Could you check a few things on this model? Use its own coordinates, in mm. Coordinates: 2 decimals unless noted, no trailing zeros. Order: outer loops, then holes, each group sorted by start corner. A loop starts at its lowest first (then second) coordinate and runs counter-clockwise, first axis right, second up. Notation, with made-up numbers: (79, -18.5) - (107, -18.5) arc R20 ccw to (107, 20.5) - close; hole circle Ø8 at (53.25, 63). An arc over 180 degrees is marked (long way). One line per item, written item: value.
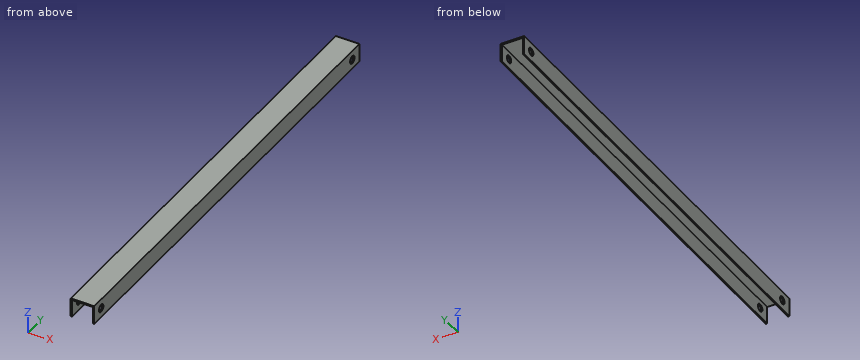
from build123d import *

# Parameters (mm, degrees)
BOSS_EXTRUDE1_DEPTH      = 145
BOSS_EXTRUDE1_DEPTH_BACK = 145
SKETCH1_W                = 15
SKETCH1_H                = 12
CUT_EXTRUDE1_DEPTH       = 200
CUT_EXTRUDE1_DEPTH_BACK  = 200
SKETCH2_W                = 13.28
SKETCH2_H                = 14
CUT_EXTRUDE2_DEPTH       = 200
CUT_EXTRUDE2_DEPTH_BACK  = 200
SKETCH3_R                = 2.4


with BuildPart() as part:
    # Sketch1 → Boss-Extrude1 (new, two sides: drawn at the far end of the back side and taken through both)
    with BuildSketch(Plane(origin=(0, 0, 0), x_dir=(1, 0, 0), z_dir=(0, 1, 0)).offset(-BOSS_EXTRUDE1_DEPTH_BACK)):
        Rectangle(SKETCH1_W, SKETCH1_H)
    extrude(amount=BOSS_EXTRUDE1_DEPTH + BOSS_EXTRUDE1_DEPTH_BACK)

    # Sketch2 → Cut-Extrude1 (cut, two sides: drawn at the far end of the back side and taken through both)
    with BuildSketch(Plane(origin=(0, 0, 0), x_dir=(1, 0, 0), z_dir=(0, 1, 0)).offset(-CUT_EXTRUDE1_DEPTH_BACK)):
        with Locations((0, 1.86)):
            Rectangle(SKETCH2_W, SKETCH2_H)
    extrude(amount=CUT_EXTRUDE1_DEPTH + CUT_EXTRUDE1_DEPTH_BACK, mode=Mode.SUBTRACT)

    # Sketch3 → Cut-Extrude2 (cut, two sides: drawn at the far end of the back side and taken through both)
    with BuildSketch(Plane(origin=(0, 0, 0), x_dir=(0, 0, -1), z_dir=(1, 0, 0)).offset(-CUT_EXTRUDE2_DEPTH_BACK)):
        with Locations(Location((0, 137.33, 0), (0, 0, 180))):
            Circle(SKETCH3_R)
        with Locations(Location((0, -137.33, 0), (0, 0, 180))):
            Circle(SKETCH3_R)
    extrude(amount=CUT_EXTRUDE2_DEPTH + CUT_EXTRUDE2_DEPTH_BACK, mode=Mode.SUBTRACT)


solid = part.part
Item 1: I want a section at C-C on x = -1.75. Please give me the cut outline in (y, z).
Conclusion:
outline: (-145, 5.14) - (145, 5.14) - (145, 6) - (-145, 6) - close
Item 2: I want a section at B-B on z = 0. Please give me the cut outline in (x, y).
Conclusion:
outline: (-7.5, -145) - (-6.64, -145) - (-6.64, -139.73) - (-7.5, -139.73) - close; (-7.5, -134.93) - (-6.64, -134.93) - (-6.64, 134.93) - (-7.5, 134.93) - close; (-7.5, 139.73) - (-6.64, 139.73) - (-6.64, 145) - (-7.5, 145) - close; (6.64, -145) - (7.5, -145) - (7.5, -139.73) - (6.64, -139.73) - close; (6.64, -134.93) - (7.5, -134.93) - (7.5, 134.93) - (6.64, 134.93) - close; (6.64, 139.73) - (7.5, 139.73) - (7.5, 145) - (6.64, 145) - close
Item 3: I want a section at A-A on y = -137.33. Please give me the cut outline in (x, z), then the cut area to 3 significant figures.
Conclusion:
outline: (-7.5, -6) - (-6.64, -6) - (-6.64, -2.4) - (-7.5, -2.4) - close; (-7.5, 2.4) - (-6.64, 2.4) - (-6.64, 5.14) - (6.64, 5.14) - (6.64, 2.4) - (7.5, 2.4) - (7.5, 6) - (-7.5, 6) - close; (6.64, -6) - (7.5, -6) - (7.5, -2.4) - (6.64, -2.4) - close
area: 23.8 mm²
Item 4: If I drill on probe 1 along Y at (x, z) = (-7.1, 0); probe 2 along Z at (x, y) = (-7.1, 137.33); probe 3 along X at (y, z) = (-29.5, 2.5), over which ranges is the centre line in solid material (lowest first)?
Conclusion:
probe 1: -145 to -139.73, -134.93 to 134.93, 139.73 to 145
probe 2: -6 to -2.4, 2.4 to 6
probe 3: -7.5 to -6.64, 6.64 to 7.5
